Drawing for the job (mm, zero at the part's lowest x, y, z). A direction names the side the tool comes from. Give positions to 0.01 mm unless a question says otherwise; leave off trailing zeros. Write each loop counter-clockwise with the first axis right and the second up, starting at its lowest first coordinate (ties: lowest second). Pieces come first, ordered by that corner, then holes. Notation, with made-up numbers: M 54,33.25 L 85,33.25 A35 ccw 85,72.25 Z; hole C -9,65 d4. An arc over 180 degrees is marked long. Use a Markdown table: item, result. Add a question column.
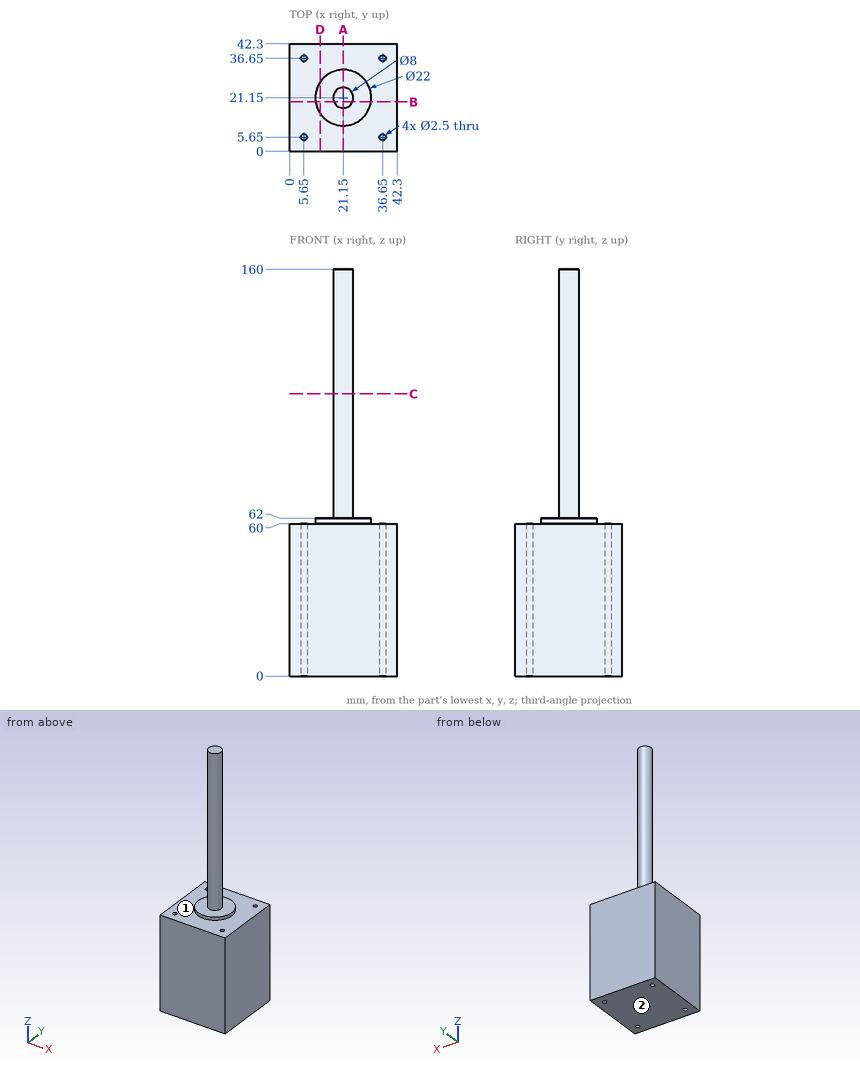
1. Flat gauge pins, fed straight in: pin 1 (2 mm diameter, centred on x = 36.65, y = 5.65, fed in from -Z); pin 2 (1.5 mm diameter, centred on x = 23.5, z = 68, fed in from -Y); pin 3 (1 mm diameter, centred on x = 10, y = 23.5, fed in from +Z); pin 4 (3 mm diameter, centred on x = 5.65, y = 5.65, fed in from +Z). Where does each tip first touch, or does it go through?
2. Drill centre lines: probe 1 along X at (y, z) = (5.5, 35.5); probe 2 along Y at (x, z) = (36.65, 13.5); probe 3 along Y at (x, z) = (36, 30). Where is each one in solid material? Low to high. Write a range as [from, to].
3. Cut at A-A (x = 21.15). Write the cut outline in (y, z).
4. Cut at D-D (x = 12). Write the cut outline in (y, z).
5. Cut at C-C (z = 111). Write the cut outline in (x, y).
6. Cut at B-B (y = 19.5). Write the cut outline in (x, z).
7. Tool access for the marked faces 1 and 2: list every direction of +Z, -Z, +X, -X, +Y, -Y with a clear straight run to the whole face (end or side of a thin tool).
A:
| question | item | result |
|---|---|---|
| 1 | pin 1 | passes through |
| 1 | pin 2 | stops at y = 17.48 |
| 1 | pin 3 | stops at z = 62 |
| 1 | pin 4 | stops at z = 60 |
| 2 | probe 1 | x = [0, 4.41], [6.89, 35.41], [37.89, 42.3] |
| 2 | probe 2 | y = [0, 4.4], [6.9, 35.4], [37.9, 42.3] |
| 2 | probe 3 | y = [0, 4.58], [6.72, 35.58], [37.72, 42.3] |
| 3 | outline | M 0,0 L 42.3,0 L 42.3,60 L 32.15,60 L 32.15,62 L 25.15,62 L 25.15,160 L 17.15,160 L 17.15,62 L 10.15,62 L 10.15,60 L 0,60 Z |
| 4 | outline | M 0,0 L 42.3,0 L 42.3,60 L 27.26,60 L 27.26,62 L 15.04,62 L 15.04,60 L 0,60 Z |
| 5 | outline | C 21.15,21.15 d8 |
| 6 | outline | M 0,0 L 42.3,0 L 42.3,60 L 32.03,60 L 32.03,62 L 24.79,62 L 24.79,160 L 17.51,160 L 17.51,62 L 10.27,62 L 10.27,60 L 0,60 Z |
| 7 | face 1 | +Z |
| 7 | face 2 | -Z, +X, -X, +Y, -Y |
